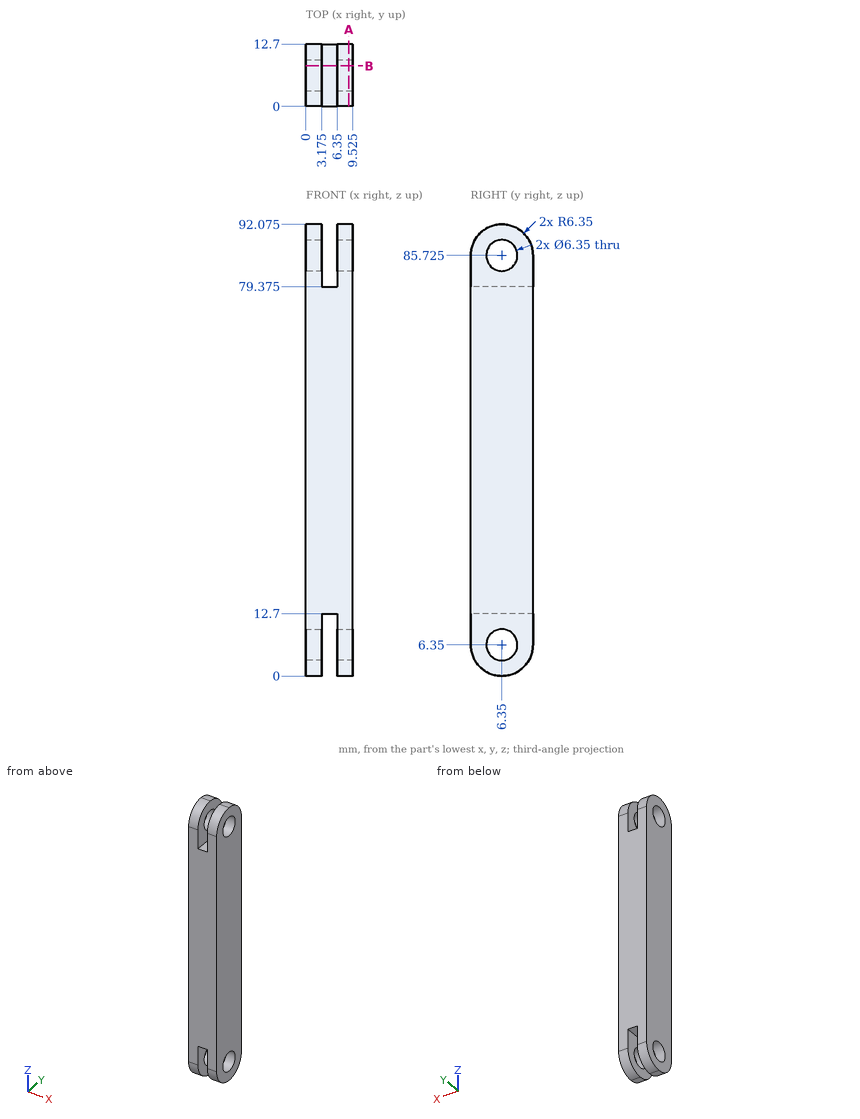
Drawing for the job (mm, zero at the part's lowest x, y, z). Coordinates: 2 decimals unless noted, no trailing zeros. Order: outer loops, then holes, each group sorted by start corner. A loop starts at its lowest first (then second) coordinate and runs counter-clockwise, first axis right, second up.
Item 1: Pin check, flat tips, straight feed: pin 1 Ø5 at (x, y) = (4, 9) entering from -Z; pin 2 Ø4 at (y, z) = (5.5, 5) entering from +X (3 decimals); pin 3 Ø1 at (x, y) = (5, 9) entering from -Z. Stop position of each tip, or through.
Check sheet entries:
pin 1: stops at z = 0.01
pin 2: stops at x = 9.525
pin 3: stops at z = 12.7
Item 2: Band-saw the part on B-B on y = 8.25. List the corners of the cut face in (x, z) (3 decimals), plus the area to 3 significant figures.
Check sheet entries:
outline: (0, 0.291) - (3.175, 0.291) - (3.175, 3.806) - (0, 3.806) - close; (0, 8.894) - (3.175, 8.894) - (3.175, 12.7) - (6.35, 12.7) - (6.35, 8.894) - (9.525, 8.894) - (9.525, 83.181) - (6.35, 83.181) - (6.35, 79.375) - (3.175, 79.375) - (3.175, 83.181) - (0, 83.181) - close; (0, 88.269) - (3.175, 88.269) - (3.175, 91.784) - (0, 91.784) - close; (6.35, 0.291) - (9.525, 0.291) - (9.525, 3.806) - (6.35, 3.806) - close; (6.35, 88.269) - (9.525, 88.269) - (9.525, 91.784) - (6.35, 91.784) - close
area: 728 mm2
Item 3: Drill centre lines: L1, parallel to X at y = 12, z = 83 (3 decimals); L2, parallel to Z at x = 3.75, y = 2 (3 decimals); L3, parallel to Y at x = 2, z = 9. Where is each one in solid material? Low to high.
Check sheet entries:
L1: x = 0 to 3.175, 6.35 to 9.525
L2: z = 12.7 to 79.375
L3: y = 0 to 4.6, 8.1 to 12.7
Item 4: Band-saw the part on A-A on x = 8.75. List the corners of the cut face in (y, z) (3 decimals), plus the area to 3 significant figures.
Check sheet entries:
outline: (0, 6.35) arc R6.35 ccw to (12.7, 6.35) - (12.7, 85.725) arc R6.35 ccw to (0, 85.725) - close; hole circle Ø6.35 at (6.35, 6.35); hole circle Ø6.35 at (6.35, 85.725)
area: 1,070 mm2
